from build123d import *

# Parameters (mm, degrees)
AUFSATZ_LINEAR_AUSTRAGEN1_DEPTH      = 3
F_3_2_3_2_DURCHMESSER_BOHRUNG1_D     = 3.2
F_3_2_3_2_DURCHMESSER_BOHRUNG1_DEPTH = 8.5
F_3_2_3_2_DURCHMESSER_BOHRUNG1_TIP   = 0.96137699


with BuildPart() as part:
    # Skizze1 → Aufsatz-Linear austragen1 (new body)
    with BuildSketch(Plane.XY):
        Polygon((-10, 70), (-54.472280452, 17), (-60, 17), (-60, 0), (0, 0), (0, 125), (-10, 125), align=None)
        Polygon((-10, 54.442761731), (-41.418207559, 17), (-10, 17), align=None, mode=Mode.SUBTRACT)
    extrude(amount=AUFSATZ_LINEAR_AUSTRAGEN1_DEPTH)

    # Ø3.2 (3.2) Durchmesser Bohrung1
    with Locations(Plane.XY.offset(3)):
        with Locations((-5, 115), (-5, 105)):
            Hole(F_3_2_3_2_DURCHMESSER_BOHRUNG1_D / 2, depth=F_3_2_3_2_DURCHMESSER_BOHRUNG1_DEPTH)
            with Locations((0, 0, -(F_3_2_3_2_DURCHMESSER_BOHRUNG1_DEPTH + F_3_2_3_2_DURCHMESSER_BOHRUNG1_TIP / 2))):  # 118° drill point
                Cone(0, F_3_2_3_2_DURCHMESSER_BOHRUNG1_D / 2, F_3_2_3_2_DURCHMESSER_BOHRUNG1_TIP, mode=Mode.SUBTRACT)


solid = part.part
Design review of the part built by this model. Coordinates are the model's own, in mm. A direction names the side the tool comes from. Round coordinates to 2 decimals unless told otherwise and drop trailing zeros. Write each loop counter-clockwise with the first axis right and the second up, starting at its lowest first coordinate (ties: lowest second). Pieces come first, ordered by that corner, then holes. Notation, with made-up numbers: (77, -24) - (81, -24) arc R7 ccw to (81, -20) - close; hole circle Ø1 at (14, -22.5). An arc over 180 degrees is marked (long way). Use a Markdown table: item, result. Add a question column.
1. For faces 1 (the face through (-57, 17, 1)), 2 (the face through (-30, 0, 1)), 3 (the face through (-26, 17, 1)), list the 3-axis set-ups (+Z, -Z, +X, -X, +Y, -Y) from which the entire face can be reached by the end or side of a thin tool; tool diameter is ignored.
2. We need section D-D (x = -18.5). State the section outline as (y, z) points, then the cut area to 3 significant figures.
3. We need section A-A (x = -5). State the section outline as (y, z) points.
4. We need section B-B (y = 115). State the section outline as (x, z) points.
5. Wall thickness on probe 1 along Y at (x, z) = (-5, 2.25); probe 2 along X at (y, z) = (115, 1); probe 3 along Y at (x, z) = (-26, 0.8): over which ranges is each line inside the solid? List them lowest first.
6. We need section C-C (z = 2). State the section outline as (x, y) points, then the cut area to 3 significant figures.
7. Mouldability with a two-part tool opening along X and no side actions: class faces 4 (the face through (-26, 40, 3)), 5 (the face through (-10, 98, 1)), 6 (the face through (-4.792, 116.586, 1.479)) as +X half, -X half, draft (parallel to the pull), parting line (faces both ways), or undercut.
8. Clearance check with flat-ended pins moving along their axes: pin 1 (2.5 mm diameter, centred on x = -5, y = 115, fed in from -Z); pin 2 (0.9 mm diameter, centred on x = -56, z = 1.5, fed in from +Y); pin 3 (1.5 mm diameter, centred on y = 74.5, z = 1.5, fed in from -X); pin 4 (5 mm diameter, centred on x = -11, y = 103.5, fed in from +Z). State where each tip first meets the part, or that it passes through.
Output:
| question | item | result |
|---|---|---|
| 1 | face 1 | +Z, -Z, -X, +Y |
| 1 | face 2 | +Z, -Z, +X, -X, -Y |
| 1 | face 3 | +Z, -Z |
| 2 | outline | (0, 0) - (17, 0) - (17, 3) - (0, 3) - close; (44.31, 0) - (59.87, 0) - (59.87, 3) - (44.31, 3) - close |
| 2 | area | 97.7 mm2 |
| 3 | outline | (0, 0) - (103.4, 0) - (103.4, 3) - (0, 3) - close; (106.6, 0) - (113.4, 0) - (113.4, 3) - (106.6, 3) - close; (116.6, 0) - (125, 0) - (125, 3) - (116.6, 3) - close |
| 4 | outline | (-10, 0) - (-6.6, 0) - (-6.6, 3) - (-10, 3) - close; (-3.4, 0) - (0, 0) - (0, 3) - (-3.4, 3) - close |
| 5 | probe 1 | y = 0 to 103.4, 106.6 to 113.4, 116.6 to 125 |
| 5 | probe 2 | x = -10 to -6.6, -3.4 to 0 |
| 5 | probe 3 | y = 0 to 17, 35.37 to 50.93 |
| 6 | outline | (-60, 0) - (0, 0) - (0, 125) - (-10, 125) - (-10, 70) - (-54.47, 17) - (-60, 17) - close; hole (-41.42, 17) - (-10, 17) - (-10, 54.44) - close; hole circle Ø3.2 at (-5, 105); hole circle Ø3.2 at (-5, 115) |
| 6 | area | 2,670 mm2 |
| 7 | face 4 | draft |
| 7 | face 5 | -X half |
| 7 | face 6 | undercut |
| 8 | pin 1 | passes through |
| 8 | pin 2 | stops at y = 17 |
| 8 | pin 3 | stops at x = -10 |
| 8 | pin 4 | stops at z = 3 |
